from build123d import *

# Parameters (mm, degrees)
F0_W     = 114
F0_H     = 195
F1_DEPTH = 55
F2_W     = 30
F2_H     = 37
F3_DEPTH = 125
F5_DEPTH = 11
F7_DEPTH = 65
F9_DEPTH = 105


with BuildPart() as f1:
    # F0 (on Top) → F1 (new body)
    with BuildSketch(Plane.XY):
        Rectangle(F0_W, F0_H)
    extrude(amount=F1_DEPTH)

    # F2 (on face) → F3 (join)
    with BuildSketch(Plane.XY.offset(55)):
        with Locations((-1, 54)):
            Rectangle(F2_W, F2_H)
    extrude(amount=F3_DEPTH)

    # F4 (on face) → F5 (join)
    with BuildSketch(Plane.XY.offset(180)):
        Polygon((14, 35.5), (-1, 35.5), (-16, 35.5), (-33.5, 35.5), (-33.5, -69.5), (-1, -69.5), (31.5, -69.5), (31.5, 35.5), align=None)
    extrude(amount=-F5_DEPTH)

    # F6 (on face) → F7 (join, through all)
    with BuildSketch(Plane.YZ.offset(31.5)):
        Polygon((-17, 232.5), (-69.5, 180), (20.5, 180), (20.5, 195), align=None)
    extrude(amount=-F7_DEPTH)

    # F8 (on face) → F9 (join)
    with BuildSketch(Plane(origin=(0, -124.75, 124.75), x_dir=(1, 0, 0), z_dir=(0, -0.707107, 0.707107))):
        Polygon((-51, 83.135299), (-33.5, 83.135299), (0, 83.135299), (33.5, 83.135299), (51, 83.135299), (51, 138.135299), (0, 138.135299), (-51, 138.135299), align=None)
    extrude(amount=F9_DEPTH)


solid = f1.part
Model file for the job. Use its own axes, mm. A direction names the side the tool comes from. Coordinates: 2 decimals unless noted, no trailing zeros. Loops run counter-clockwise (first coordinate to the right, second up) from the corner with the lowest first, then second, coordinate; pieces in that order, holes last. Notation, with made-up numbers: (1.5, 37) -> (25.5, 37) arc R8 cw to (25.5, 49) -> close; hole circle Ø5 at (-39, -21.5). An arc over 180 degrees is marked (long way). Use one line per item in the form item = value. Start each with the question number.
(1) Cut at D-D on x = 1. Give the cut face in (y, z), and give its area (3 significant figures).
(2) Flat gauge pins, fed straight in: pin 1 (12 mm diameter, centred on y = -77, z = 213.5, fed in from -X); pin 2 (12 mm diameter, centred on x = -19.5, y = 34, fed in from +Z); pin 3 (6 mm diameter, centred on x = 8.5, z = 57, fed in from -Y). Where does each tip first touch, or does it go through?
(3) Tool access for faces 1 (the flat face through (-25, 35.5, 175)), 2 (the flat face through (-1, -97.5, 27)), 3 (the flat face through (-1, -69.5, 175)), 4 (the flat face through (-0.5, -22, 227.5)), 5 (the flat face through (-42.4, -46.2, 203.3)): list every direction of +Z, -Z, +X, -X, +Y, -Y with a clear straight run to the whole face (end or side of a thin tool).
(4) Cut at A-A on x = 23. Give the cut face in (y, z).
(5) Cut at C-C on y = -6.5. Give the cut face in (x, z).
(6) Pull direction Z, two halves, no side cores. Call faces 6 (the flat face through (-1, 1, 0)), 7 (the flat face through (-0.71, -102.57, 220.14)), 8 (the flat face through (-1, 35.5, 111)), 9 (the flat face through (-51, -83, 240)): pulls with the +Z half, pulls with the -Z half, needs draft (parallel to the pull), parting line crosses it, or undercut.
(7) Probe probe 1 along Z at (x, y) = (42, 77.5); probe 2 along Y at (x, z) = (39.5, 39.5); probe 3 along Y at (x, z) = (13, 64.5). List the from-to ranges inside material, lowest first. Write a range as from..to.
(8) Cut at B-B on y = 52.5. Give the cut face in (x, z).
Values:
q1.outline = (-140.21, 257.78) -> (-65.96, 183.54) -> (-69.5, 180) -> (-69.5, 169) -> (35.5, 169) -> (35.5, 55) -> (-97.5, 55) -> (-97.5, 0) -> (97.5, 0) -> (97.5, 55) -> (72.5, 55) -> (72.5, 180) -> (20.5, 180) -> (20.5, 195) -> (-17, 232.5) -> (-27.07, 222.43) -> (-101.32, 296.67) -> close
q1.area = 24,900 mm2
q2.pin_1 = -51
q2.pin_2 = 180
q2.pin_3 = -97.5
q3.face_1 = +Z, -X, +Y
q3.face_2 = -Z, +X, -X, -Y
q3.face_3 = +X, -X, -Y
q3.face_4 = +Z, +X, -X
q3.face_5 = -X, +Y
q4.outline = (-140.21, 257.78) -> (-65.96, 183.54) -> (-69.5, 180) -> (-69.5, 169) -> (35.5, 169) -> (35.5, 180) -> (20.5, 180) -> (20.5, 195) -> (-17, 232.5) -> (-27.07, 222.43) -> (-101.32, 296.67) -> close; (-97.5, 0) -> (97.5, 0) -> (97.5, 55) -> (-97.5, 55) -> close
q5.outline = (-57, 0) -> (57, 0) -> (57, 55) -> (-57, 55) -> close; (-33.5, 169) -> (31.5, 169) -> (31.5, 222) -> (-33.5, 222) -> close
q6.face_6 = pulls with the -Z half
q6.face_7 = undercut
q6.face_8 = undercut
q6.face_9 = needs draft
q7.probe_1 = 0..55
q7.probe_2 = -97.5..97.5
q7.probe_3 = 35.5..72.5
q8.outline = (-57, 0) -> (57, 0) -> (57, 55) -> (14, 55) -> (14, 180) -> (-16, 180) -> (-16, 55) -> (-57, 55) -> close
